```python
from build123d import *

# Parameters (mm, degrees)
EXTRUDE_THIN1_DEPTH      = 12.7
EXTRUDE_THIN1_DEPTH_BACK = 12.7
CUT_EXTRUDE1_DEPTH       = 4.7625
CUT_EXTRUDE2_REACH       = 146.244
SKETCH3_R                = 6.35


with BuildPart() as part:
    # Sketch1 → Extrude-Thin1 (new, two sides: drawn at the far end of the back side and taken through both)
    with BuildSketch(Plane.XY.offset(-EXTRUDE_THIN1_DEPTH_BACK)):
        with BuildLine():
            Line((0, 101.6), (0, 25.4))
            ThreePointArc((0, 25.4), (7.439487758, 7.439487758), (25.4, 0))
            Line((25.4, 0), (101.6, 0))
            Line((101.6, 0), (101.6, -4.7625))
            Line((101.6, -4.7625), (25.4, -4.7625))
            ThreePointArc((25.4, -4.7625), (4.071891712, 4.071891712), (-4.7625, 25.4))
            Line((-4.7625, 25.4), (-4.7625, 101.6))
            Line((-4.7625, 101.6), (0, 101.6))
        make_face()
    extrude(amount=EXTRUDE_THIN1_DEPTH + EXTRUDE_THIN1_DEPTH_BACK)

    # Sketch2 → Cut-Extrude1 (cut)
    with BuildSketch(Plane(origin=(0, 0, 0), x_dir=(-1, 0, 0), z_dir=(0, 1, 0))):
        with BuildLine():
            Line((-88.9, 12.7), (-88.9, 23.152683053))
            Line((-88.9, 23.152683053), (-107.491491885, 23.152683053))
            Line((-107.491491885, 23.152683053), (-107.491491885, -20.225178662))
            Line((-107.491491885, -20.225178662), (-88.9, -20.225178662))
            Line((-88.9, -20.225178662), (-88.9, -12.7))
            ThreePointArc((-88.9, -12.7), (-101.6, 0), (-88.9, 12.7))
        make_face()
    extrude(amount=-CUT_EXTRUDE1_DEPTH, mode=Mode.SUBTRACT)

    # Sketch3 → Cut-Extrude2 (cut, up to next)
    with BuildSketch(Plane(origin=(0, 0, 0), x_dir=(0, 0, -1), z_dir=(1, 0, 0)), mode=Mode.PRIVATE) as cut_extrude2_sk1:
        with Locations(Location((0, 63.5, 0), (0, 0, 90))):
            Circle(SKETCH3_R)
    cut_extrude2_tool1 = extrude(cut_extrude2_sk1.sketch, amount=-CUT_EXTRUDE2_REACH, mode=Mode.PRIVATE) & part.part
    add(cut_extrude2_tool1.solids().sort_by_distance((0, 63.5, 0))[0], mode=Mode.SUBTRACT)


solid = part.part
```
Geometry check sheet. Reference: the model listing, model coordinates, mm. A direction names the side the tool comes from. Coordinates: 2 decimals unless noted, no trailing zeros. Loops run counter-clockwise (first coordinate to the right, second up) from the corner with the lowest first, then second, coordinate; pieces in that order, holes last. Notation, with made-up numbers: (-1.5, 29.5) - (28.5, 29.5) arc R32 ccw to (28.5, 67.5) - close; hole circle Ø8 at (-20, 39). An arc over 180 degrees is marked (long way). One line per item, written item: value. Start each with the question number.
(1) Cross-section at C-C on x = 33.5. Enter the section's corners in (y, z).
(2) Tool access check on faces 1 (the flat face through (1, 17, -12.7)), 2 (the flat face through (0, 56, 0)). Record the directions out of +Z, -Z, +X, -X, +Y, -Y that give a thin tool (end or side, any length) a straight path to the whole face; none if there is none.
(3) Material ranges on line 1 (Z direction, x = -1.25, y = 63.5); line 2 (Y direction, x = 53.5, z = 7.5), recorded low to high. Write a range as [from, to].
(4) Cross-section at D-D on z = 8.5. Enter the section's corners in (x, y) (1 decimal).
(5) Mould release check, pull along Y, two halves, no side actions. Record for faces 3 (the flat face through (-2, 101.6, 0)), 4 (the cylindrical face through (-2.348, 57.156, 0.279)), 5 (the flat face through (1, 17, 12.7)): released by +Y, released by -Y, zero draft, split by the parting line, or undercut.
(6) Depth check by flat-ended pin: P1, Ø2, axis at y = 47, z = 0, coming from the +X side; P2, Ø14.5, axis at y = 63.5, z = 0, coming from the -X side; P3, Ø12.5, axis at x = 79, z = 6, coming from the +Y side; P4, Ø1.5, axis at y = 21, z = -3, coming from the +X side. Enter the tip coordinate at first touch or a pass-through.
(7) Cross-section at B-B on y = 63.5. Enter the section's corners in (x, z), plus the area to 3 significant figures.
Results below:
1. outline: (-4.76, -12.7) - (0, -12.7) - (0, 12.7) - (-4.76, 12.7) - close
2. face 1: -Z, +X, -X, +Y, -Y
2. face 2: +Z, -Z, +X, +Y
3. line 1: z = [-12.7, -6.35], [6.35, 12.7]
3. line 2: y = [-4.76, 0]
4. outline: (-4.8, 25.4) arc R30.2 ccw to (25.4, -4.8) - (98.3, -4.8) - (98.3, 0) - (25.4, 0) arc R25.4 cw to (0, 25.4) - (0, 101.6) - (-4.8, 101.6) - close
5. face 3: released by +Y
5. face 4: undercut
5. face 5: zero draft
6. P1: stops at x = 0
6. P2: stops at x = -4.76
6. P3: stops at y = 0
6. P4: stops at x = 0.53
7. outline: (-4.76, -12.7) - (0, -12.7) - (0, -6.35) - (-4.76, -6.35) - close; (-4.76, 6.35) - (0, 6.35) - (0, 12.7) - (-4.76, 12.7) - close
7. area: 60.5 mm2
